Verification items for this drawing (mm, ordinates from the low corner). Give positions to 0.01 mm unless a question says otherwise; leave off trailing zeros. Order: outer loops, then holes, each group sorted by start corner. A loop starts at its lowest first (then second) coordinate and runs counter-clockwise, first axis right, second up.
(1) Sectioned sample at C-C on x = 27. Record the cut outline in (y, z), plus the area to 3 significant figures.
(2) Sectioned sample at B-B on y = 42.5. Record the cut outline in (x, z), plus the area to 3 significant figures.
(3) Gauge pin test, flat ends, axial feed: pin 1 (0.9 mm diameter, centred on y = 248.5, z = 2, fed in from -X); pin 2 (1.5 mm diameter, centred on x = 204.5, z = 1, fed in from +Y); pin 3 (0.9 mm diameter, centred on x = 185.5, z = 1.5, fed in from -Y). Record the tip position at first contact, or that the pin passes through.
(4) Scan lines: L1, parallel to Y at x = 38, z = 1.8; L2, parallel to X at y = 67.5, z = 2.6. Record each from-to range of solid material in increasing order.
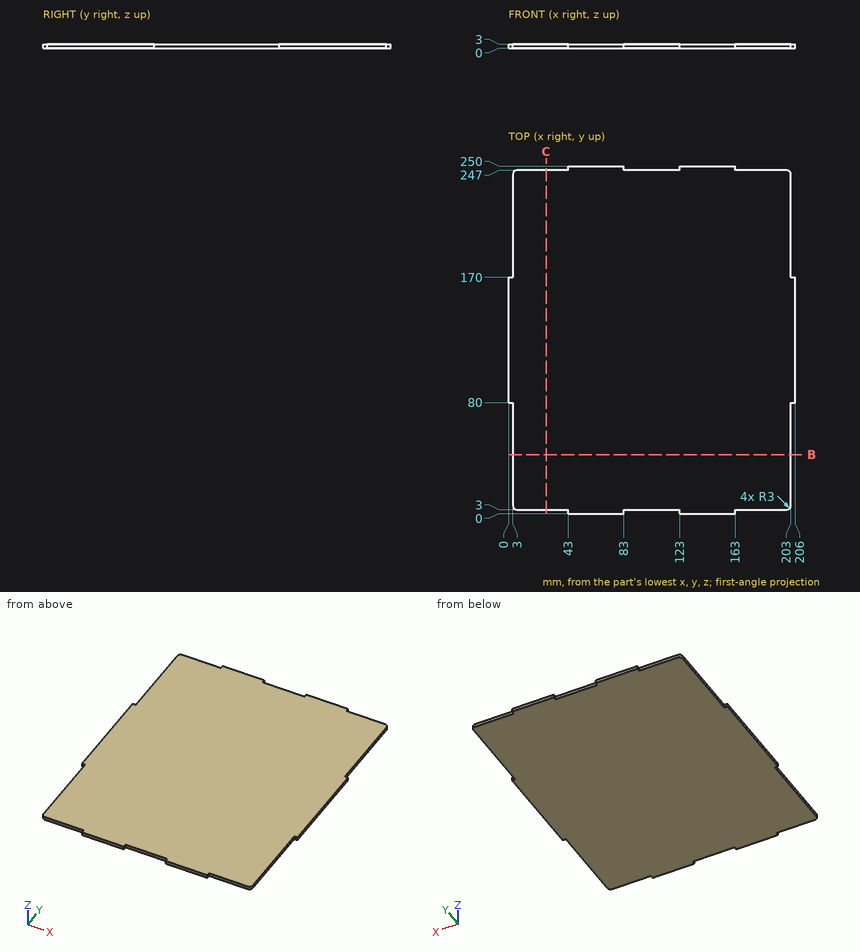
Ans:
1. outline: (3, 0) - (247, 0) - (247, 3) - (3, 3) - close
1. area: 732 mm2
2. outline: (3, 0) - (203, 0) - (203, 3) - (3, 3) - close
2. area: 600 mm2
3. pin 1: stops at x = 43
3. pin 2: stops at y = 170
3. pin 3: stops at y = 3
4. L1: y = 3 to 247
4. L2: x = 3 to 203
